The listing builds one solid part. Answer for the finished solid, in the listing's coordinates (mm). Face numbers are marked on the shaded views. A direction names the side the tool comes from. Round coordinates to 2 decimals unless told otherwise and drop trailing zeros. Order: outer loops, then holes, each group sorted by start corner. A loop starts at its lowest first (then second) coordinate and runs counter-clockwise, first axis right, second up. Notation, with made-up numbers: (-27, 51.5) - (30, 51.5) arc R17 ccw to (30, 58.5) - close; hole circle Ø1 at (-4, 44.5). An arc over 180 degrees is marked (long way). Write item = value, one per line.
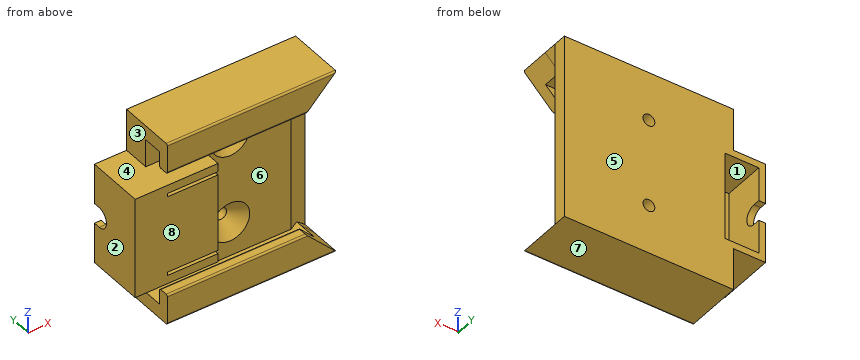
from build123d import *

# Parameters (mm, degrees)
SKETCH_1_W          = 50
SKETCH_1_H          = 55
EXTRUDE_1_DEPTH     = 6
SKETCH_2_W          = 15
SKETCH_2_H          = 30
EXTRUDE_2_DEPTH     = 9
SKETCH_3_W          = 15
SKETCH_3_H          = 1
CUT_EXTRUDE_1_DEPTH = 7
SKETCH_4_W          = 50
SKETCH_4_H          = 4.25
EXTRUDE_3_DEPTH     = 9.5
SKETCH_5_W          = 50
SKETCH_5_H          = 3.7
EXTRUDE_4_DEPTH     = 4.75
CUT_EXTRUDE_2_DEPTH = 9.5
SKETCH_7_W          = 30
SKETCH_7_H          = 15
EXTRUDE_5_DEPTH     = 9.5
SKETCH_8_W          = 10
SKETCH_8_H          = 26
CUT_EXTRUDE_3_DEPTH = 10.5
SKETCH_9_R          = 3
CUT_EXTRUDE_4_DEPTH = 7.5
SKETCH_10_R         = 1.75
CUT_EXTRUDE_5_DEPTH = 7.5
CHAMFER_1_SIZE      = 4
SKETCH_11_R         = 1.75
EXTRUDE_6_DEPTH     = 2
SKETCH_12_W         = 89.739519214
SKETCH_12_H         = 69.095216672
CUT_EXTRUDE_6_DEPTH = 0.5
CHAMFER_2_SIZE      = 7
CHAMFER_2_SIZE_2    = 4.041451884
FILLET_1_R          = 0.5


with BuildPart() as part:
    # Эскиз1 → Бобышка-Вытянуть1 (new body)
    with BuildSketch(Plane(origin=(0, 0, 0), x_dir=(1, 0, 0), z_dir=(0, 1, 0))):
        Rectangle(SKETCH_1_W, SKETCH_1_H)
    extrude(amount=EXTRUDE_1_DEPTH)

    # Эскиз2 → Бобышка-Вытянуть2 (add)
    with BuildSketch(Plane.XZ):
        with Locations((-17.5, 0)):
            Rectangle(SKETCH_2_W, SKETCH_2_H)
    extrude(amount=EXTRUDE_2_DEPTH)

    # Эскиз3 → Вырез-Вытянуть1 (cut)
    with BuildSketch(Plane.XZ.offset(9)):
        with Locations((-17.5, 12)):
            Rectangle(SKETCH_3_W, SKETCH_3_H)
        with Locations((-17.5, -12)):
            Rectangle(SKETCH_3_W, SKETCH_3_H)
    extrude(amount=-CUT_EXTRUDE_1_DEPTH, mode=Mode.SUBTRACT)

    # Эскиз4 → Бобышка-Вытянуть3 (add)
    with BuildSketch(Plane.XZ):
        with Locations((0, -25.375)):
            Rectangle(SKETCH_4_W, SKETCH_4_H)
        with Locations((0, 25.375)):
            Rectangle(SKETCH_4_W, SKETCH_4_H)
    extrude(amount=EXTRUDE_3_DEPTH)

    # Эскиз5 → Бобышка-Вытянуть4 (add)
    with BuildSketch(Plane(origin=(0, 0, 23.25), x_dir=(-1, 0, 0), z_dir=(0, 0, -1))):
        with Locations((0, -7.65)):
            Rectangle(SKETCH_5_W, SKETCH_5_H)
    extrude_4 = extrude(amount=EXTRUDE_4_DEPTH)

    # Зеркальное отражение1: Бобышка-Вытянуть4 across plane
    add(extrude_4.mirror(Plane.XY))

    # Эскиз6 → Вырез-Вытянуть2 (cut)
    with BuildSketch(Plane.XZ):
        Polygon((16.087749561, -18.5), (25, -27.5), (25, -18.5), align=None)
        Polygon((25, 18.5), (16.087749561, 18.5), (25, 27.5), align=None)
    extrude(amount=CUT_EXTRUDE_2_DEPTH, mode=Mode.SUBTRACT)

    # Эскиз7 → Бобышка-Вытянуть5 (add)
    with BuildSketch(Plane.ZY.offset(25)):
        with Locations((0, -1.5)):
            Rectangle(SKETCH_7_W, SKETCH_7_H)
    extrude(amount=EXTRUDE_5_DEPTH)

    # Эскиз8 → Вырез-Вытянуть3 (cut)
    with BuildSketch(Plane(origin=(0, 6, 0), x_dir=(1, 0, 0), z_dir=(0, 1, 0))):
        with Locations((-27.5, 0)):
            Rectangle(SKETCH_8_W, SKETCH_8_H)
    extrude(amount=-CUT_EXTRUDE_3_DEPTH, mode=Mode.SUBTRACT)

    # Эскиз9 → Вырез-Вытянуть4 (cut)
    with BuildSketch(Plane.ZY.offset(34.5)):
        with Locations((0, 6)):
            Circle(SKETCH_9_R)
    extrude(amount=-CUT_EXTRUDE_4_DEPTH, mode=Mode.SUBTRACT)

    # Эскиз10 → Вырез-Вытянуть5 (cut)
    with BuildSketch(Plane.XZ):
        with Locations(Location((0, 13, 0), (0, 0, 270))):
            Circle(SKETCH_10_R)
        with Locations(Location((0, -13, 0), (0, 0, 270))):
            Circle(SKETCH_10_R)
    extrude(amount=-CUT_EXTRUDE_5_DEPTH, mode=Mode.SUBTRACT)

    # Фаска1
    chamfer_1_edges = [part.edges().sort_by_distance(p)[0] for p in [
        (0, 0, 14.75),
        (0, 0, -11.25),
    ]]
    chamfer(chamfer_1_edges, length=CHAMFER_1_SIZE)

    # Эскиз11 → Бобышка-Вытянуть6 (add)
    with BuildSketch(Plane(origin=(0, 6, 0), x_dir=(1, 0, 0), z_dir=(0, 1, 0))):
        Polygon((-34.5, 3), (-32.5, 3), (-32.5, 13), (-22.5, 13), (-22.5, -13), (-32.5, -13), (-32.5, -3), (-34.5, -3), (-34.5, -15), (-25, -15), (-25, -27.5), (25, -27.5), (25, 27.5), (-25, 27.5), (-25, 15), (-34.5, 15), align=None)
        with Locations(Location((0, 13, 0), (0, 0, 90))):
            Circle(SKETCH_11_R, mode=Mode.SUBTRACT)
        with Locations(Location((0, -13, 0), (0, 0, 90))):
            Circle(SKETCH_11_R, mode=Mode.SUBTRACT)
    extrude(amount=EXTRUDE_6_DEPTH)

    # Эскиз12 → Вырез-Вытянуть6 (cut)
    with BuildSketch(Plane.XZ.offset(9.5)):
        with Locations((1.274872697, 1.26393689)):
            Rectangle(SKETCH_12_W, SKETCH_12_H)
    extrude(amount=-CUT_EXTRUDE_6_DEPTH, mode=Mode.SUBTRACT)

    # Фаска2
    # the kernel refuses this chamfer: 7, 4.041451884 mm, written as the material it takes off along each edge
    with BuildSketch(Plane(origin=(25, 0, 45.609600283), x_dir=(-0.9998132206222079, -0.019326765612700747, 0), z_dir=(0, 0, -1))) as chamfer_2_piece_1_section:
        Polygon((CHAMFER_2_SIZE * 0.999813220622, CHAMFER_2_SIZE * 0.0193267656127), (-CHAMFER_2_SIZE_2 * 0.0193267656143, CHAMFER_2_SIZE_2 * 0.999813220703), (0, 0), align=None)
    chamfer_2_piece_1 = extrude(amount=91.219200565, mode=Mode.PRIVATE)
    chamfer_2_piece_1 = split(chamfer_2_piece_1, bisect_by=Plane(origin=(23.020268738, 1.666507019, 25.500776405), z_dir=(0.7105622702047159, 0, -0.7036343227568711)), keep=Keep.TOP, mode=Mode.PRIVATE)
    chamfer_2_piece_1 = split(chamfer_2_piece_1, bisect_by=Plane(origin=(23.772949655, 1.666507019, -23.25), z_dir=(0, 0, 1)), keep=Keep.TOP, mode=Mode.PRIVATE)
    add(chamfer_2_piece_1, mode=Mode.SUBTRACT)
    with BuildSketch(Plane(origin=(25, 0, 45.609600283), x_dir=(-0.9998132206222079, -0.019326765612700747, 0), z_dir=(0, 0, -1))) as chamfer_2_piece_2_section:
        Polygon((CHAMFER_2_SIZE * 0.999813220622, CHAMFER_2_SIZE * 0.0193267656127), (-CHAMFER_2_SIZE_2 * 0.0193267656143, CHAMFER_2_SIZE_2 * 0.999813220703), (0, 0), align=None)
    chamfer_2_piece_2 = extrude(amount=91.219200565, mode=Mode.PRIVATE)
    chamfer_2_piece_2 = split(chamfer_2_piece_2, bisect_by=Plane(origin=(-2.796120558, 0.402909268, 0.569799735), z_dir=(0.7105622702047159, 0, 0.7036343227568711)), keep=Keep.TOP, mode=Mode.PRIVATE)
    chamfer_2_piece_2 = split(chamfer_2_piece_2, bisect_by=Plane(origin=(19.395718646, 0.402909268, 23.25), z_dir=(0, 0, -1)), keep=Keep.TOP, mode=Mode.PRIVATE)
    add(chamfer_2_piece_2, mode=Mode.SUBTRACT)

    # Скругление1
    fillet_1_edges = [part.edges().sort_by_distance(p)[0] for p in [
        (0, -9, 27.5),
        (-4.45612522, -9, 18.5),
        (-4.45612522, -9, -18.5),
        (0, -9, -27.5),
        (-4.45612522, -5.8, 18.5),
        (-4.45612522, -5.8, -18.5),
    ]]
    fillet(fillet_1_edges, radius=FILLET_1_R)


solid = part.part
Q1. Section D-D on z = 0 is taken. Determine the outline of the cut face in (x, y), then the cut area to 3 significant figures.
Model answer:
outline = (-34.5, -9) - (-10, -9) - (-10, 0) - (18, 0) - (25, 4.04) - (25, 8) - (-22.5, 8) - (-22.5, -4.5) - (-32.5, -4.5) - (-32.5, 3) - (-34.5, 3) - close
area = 547 mm^2
Q2. Section A-A on x = 0 is taken. Count the separate pieces of the cut face and the enclosed holes in it, then the cut area to 3 significant figures.
Model answer:
separate_pieces = 3
enclosed_holes = 0
area = 459 mm^2
Q3. Section B-B on z = 6 is taken. Determine the outline of the cut face in (x, y).
Model answer:
outline = (-34.5, -9) - (-10, -9) - (-10, 0) - (18, 0) - (25, 4.04) - (25, 8) - (-22.5, 8) - (-22.5, -4.5) - (-32.5, -4.5) - (-32.5, 8) - (-34.5, 8) - close
Q4. For the marked faces 1, 2, 3 and 4, determine the directions among +Z, -Z, +X, -X, +Y, -Y from which every point of the face is accessible in a straight line to the end or side of a thin tool.
Model answer:
face_1 = +Y
face_2 = +Z, -Z, -X, +Y, -Y
face_3 = +Z, -X, +Y, -Y
face_4 = -X, -Y
Q5. Determine the mould class of the marked faces 5, 6, 7 and 8 for opening direction Y: released by +Y, released by -Y, zero draft, split by the parting line, or undercut.
Model answer:
face_5 = released by +Y
face_6 = undercut
face_7 = zero draft
face_8 = released by -Y
Q6. Flat-ended cylindrical pins translate along their axes: P1, Ø2, axis at x = -33.5, y = 7.5, coming from the -Z side; P2, Ø1, axis at x = -14.5, z = 17, coming from the -Y side; P3, Ø10, axis at y = 3.5, z = 23, coming from the -X side. Find the tip coordinate at first contact, or state that the pin passes through.
Model answer:
P1 = -15
P2 = 0
P3 = -25
Q7. Find the intervals of material crossed by line 1 (Z direction, x = 0, y = 7.15); line 2 (Z direction, x = 2, y = -5.25); line 3 (Y direction, x = 8, z = -20), in increasing order. Write a range as from..to.
Model answer:
line_1 = -27.5..-14.75, -11.25..11.25, 14.75..27.5
line_2 = -27.5..-23.25, 23.25..27.5
line_3 = -9..-5.8, 0..8
